CAD build for the part. Positions are in the model's coordinates, mm. Face numbers are marked on the shaded views. A direction names the side the tool comes from. Round coordinates to 2 decimals unless told otherwise and drop trailing zeros. Order: outer loops, then holes, each group sorted by start corner. A loop starts at its lowest first (then second) coordinate and runs counter-clockwise, first axis right, second up.
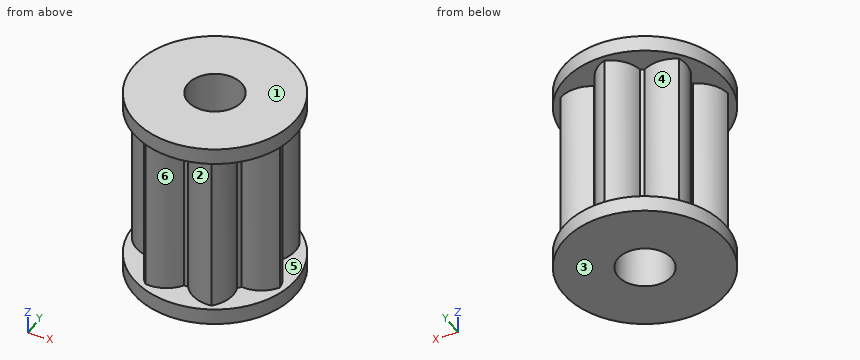
```python
from build123d import *

# Parameters (mm, degrees)
F0_R     = 2.5
F1_DEPTH = 15
F2_R     = 7.5
F2_R_2   = 2.5
F3_DEPTH = 1.5
F4_R     = 7.5
F4_R_2   = 2.5
F5_DEPTH = 1.5


with BuildPart() as f1:
    # F0 (on Top) → F1 (new body)
    with BuildSketch(Plane.XY):
        with BuildLine():
            ThreePointArc((0, 7), (-1.3412127701, 6.0735823287), (-2, 4.582575695))
            ThreePointArc((-2, 4.582575695), (-2.1694186956, 4.5048443395), (-2.3358223454, 4.420852177))
            ThreePointArc((-2.3358223454, 4.420852177), (-3.9122853917, 4.8354190111), (-5.4728203773, 4.364428613))
            ThreePointArc((-5.4728203773, 4.364428613), (-5.5847503602, 2.7382142744), (-4.8297815528, 1.2935262471))
            ThreePointArc((-4.8297815528, 1.2935262471), (-4.8746395609, 1.1126046698), (-4.9127228226, 0.9301368008))
            ThreePointArc((-4.9127228226, 0.9301368008), (-6.2197528574, -0.0439134465), (-6.8244953853, -1.5576465377))
            ThreePointArc((-6.8244953853, -1.5576465377), (-5.622857021, -2.659084978), (-4.0226390868, -2.9695748479))
            ThreePointArc((-4.0226390868, -2.9695748479), (-3.9091574123, -3.1174490093), (-3.7902428131, -3.2609905577))
            ThreePointArc((-3.7902428131, -3.2609905577), (-3.8436195617, -4.8901781832), (-3.0371861738, -6.3067820753))
            ThreePointArc((-3.0371861738, -6.3067820753), (-1.4268376596, -6.0540390065), (-0.1863673415, -4.9965255142))
            ThreePointArc((-0.1863673415, -4.9965255142), (0, -5), (0.1863673415, -4.9965255142))
            ThreePointArc((0.1863673415, -4.9965255142), (1.4268376596, -6.0540390065), (3.0371861738, -6.3067820753))
            ThreePointArc((3.0371861738, -6.3067820753), (3.8436195617, -4.8901781832), (3.7902428131, -3.2609905577))
            ThreePointArc((3.7902428131, -3.2609905577), (3.9091574123, -3.1174490093), (4.0226390868, -2.9695748479))
            ThreePointArc((4.0226390868, -2.9695748479), (5.622857021, -2.659084978), (6.8244953853, -1.5576465377))
            ThreePointArc((6.8244953853, -1.5576465377), (6.2197528574, -0.0439134465), (4.9127228226, 0.9301368008))
            ThreePointArc((4.9127228226, 0.9301368008), (4.8746395609, 1.1126046698), (4.8297815528, 1.2935262471))
            ThreePointArc((4.8297815528, 1.2935262471), (5.5847503602, 2.7382142744), (5.4728203773, 4.364428613))
            ThreePointArc((5.4728203773, 4.364428613), (3.9122853917, 4.8354190111), (2.3358223454, 4.420852177))
            ThreePointArc((2.3358223454, 4.420852177), (2.1694186956, 4.5048443395), (2, 4.582575695))
            ThreePointArc((2, 4.582575695), (1.3412127701, 6.0735823287), (0, 7))
        make_face()
        Circle(F0_R, mode=Mode.SUBTRACT)
    extrude(amount=F1_DEPTH)

    # F2 (on face) → F3 (join)
    with BuildSketch(Plane.XY.offset(15)):
        Circle(F2_R)
        with BuildLine():
            ThreePointArc((4.8297815528, 1.2935262471), (4.8746395609, 1.1126046698), (4.9127228226, 0.9301368008))
            ThreePointArc((4.9127228226, 0.9301368008), (6.2197528574, -0.0439134465), (6.8244953853, -1.5576465377))
            ThreePointArc((6.8244953853, -1.5576465377), (5.622857021, -2.659084978), (4.0226390868, -2.9695748479))
            ThreePointArc((4.0226390868, -2.9695748479), (3.9091574123, -3.1174490093), (3.7902428131, -3.2609905577))
            ThreePointArc((3.7902428131, -3.2609905577), (3.8436195617, -4.8901781832), (3.0371861738, -6.3067820753))
            ThreePointArc((3.0371861738, -6.3067820753), (1.4268376596, -6.0540390065), (0.1863673415, -4.9965255142))
            ThreePointArc((0.1863673415, -4.9965255142), (0, -5), (-0.1863673415, -4.9965255142))
            ThreePointArc((-0.1863673415, -4.9965255142), (-1.4268376596, -6.0540390065), (-3.0371861738, -6.3067820753))
            ThreePointArc((-3.0371861738, -6.3067820753), (-3.8436195617, -4.8901781832), (-3.7902428131, -3.2609905577))
            ThreePointArc((-3.7902428131, -3.2609905577), (-3.9091574123, -3.1174490093), (-4.0226390868, -2.9695748479))
            ThreePointArc((-4.0226390868, -2.9695748479), (-5.622857021, -2.659084978), (-6.8244953853, -1.5576465377))
            ThreePointArc((-6.8244953853, -1.5576465377), (-6.2197528574, -0.0439134465), (-4.9127228226, 0.9301368008))
            ThreePointArc((-4.9127228226, 0.9301368008), (-4.8746395609, 1.1126046698), (-4.8297815528, 1.2935262471))
            ThreePointArc((-4.8297815528, 1.2935262471), (-5.5847503602, 2.7382142744), (-5.4728203773, 4.364428613))
            ThreePointArc((-5.4728203773, 4.364428613), (-3.9122853917, 4.8354190111), (-2.3358223454, 4.420852177))
            ThreePointArc((-2.3358223454, 4.420852177), (-2.1694186956, 4.5048443395), (-2, 4.582575695))
            ThreePointArc((-2, 4.582575695), (-1.3412127701, 6.0735823287), (0, 7))
            ThreePointArc((0, 7), (1.3412127701, 6.0735823287), (2, 4.582575695))
            ThreePointArc((2, 4.582575695), (2.1694186956, 4.5048443395), (2.3358223454, 4.420852177))
            ThreePointArc((2.3358223454, 4.420852177), (3.9122853917, 4.8354190111), (5.4728203773, 4.364428613))
            ThreePointArc((5.4728203773, 4.364428613), (5.5847503602, 2.7382142744), (4.8297815528, 1.2935262471))
        make_face(mode=Mode.SUBTRACT)
        with BuildLine():
            ThreePointArc((6.8244953853, -1.5576465377), (6.2197528574, -0.0439134465), (4.9127228226, 0.9301368008))
            ThreePointArc((4.9127228226, 0.9301368008), (4.8746395609, 1.1126046698), (4.8297815528, 1.2935262471))
            ThreePointArc((4.8297815528, 1.2935262471), (5.5847503602, 2.7382142744), (5.4728203773, 4.364428613))
            ThreePointArc((5.4728203773, 4.364428613), (3.9122853917, 4.8354190111), (2.3358223454, 4.420852177))
            ThreePointArc((2.3358223454, 4.420852177), (2.1694186956, 4.5048443395), (2, 4.582575695))
            ThreePointArc((2, 4.582575695), (1.3412127701, 6.0735823287), (0, 7))
            ThreePointArc((0, 7), (-1.3412127701, 6.0735823287), (-2, 4.582575695))
            ThreePointArc((-2, 4.582575695), (-2.1694186956, 4.5048443395), (-2.3358223454, 4.420852177))
            ThreePointArc((-2.3358223454, 4.420852177), (-3.9122853917, 4.8354190111), (-5.4728203773, 4.364428613))
            ThreePointArc((-5.4728203773, 4.364428613), (-5.5847503602, 2.7382142744), (-4.8297815528, 1.2935262471))
            ThreePointArc((-4.8297815528, 1.2935262471), (-4.8746395609, 1.1126046698), (-4.9127228226, 0.9301368008))
            ThreePointArc((-4.9127228226, 0.9301368008), (-6.2197528574, -0.0439134465), (-6.8244953853, -1.5576465377))
            ThreePointArc((-6.8244953853, -1.5576465377), (-5.622857021, -2.659084978), (-4.0226390868, -2.9695748479))
            ThreePointArc((-4.0226390868, -2.9695748479), (-3.9091574123, -3.1174490093), (-3.7902428131, -3.2609905577))
            ThreePointArc((-3.7902428131, -3.2609905577), (-3.8436195617, -4.8901781832), (-3.0371861738, -6.3067820753))
            ThreePointArc((-3.0371861738, -6.3067820753), (-1.4268376596, -6.0540390065), (-0.1863673415, -4.9965255142))
            ThreePointArc((-0.1863673415, -4.9965255142), (0, -5), (0.1863673415, -4.9965255142))
            ThreePointArc((0.1863673415, -4.9965255142), (1.4268376596, -6.0540390065), (3.0371861738, -6.3067820753))
            ThreePointArc((3.0371861738, -6.3067820753), (3.8436195617, -4.8901781832), (3.7902428131, -3.2609905577))
            ThreePointArc((3.7902428131, -3.2609905577), (3.9091574123, -3.1174490093), (4.0226390868, -2.9695748479))
            ThreePointArc((4.0226390868, -2.9695748479), (5.622857021, -2.659084978), (6.8244953853, -1.5576465377))
        make_face()
        Circle(F2_R_2, mode=Mode.SUBTRACT)
    extrude(amount=F3_DEPTH)

    # F4 (on face) → F5 (join)
    with BuildSketch(Plane(origin=(0, 0, 0), x_dir=(1, 0, 0), z_dir=(0, 0, -1))):
        Circle(F4_R)
        with BuildLine():
            ThreePointArc((4.9127228226, -0.9301368008), (4.8746395609, -1.1126046698), (4.8297815528, -1.2935262471))
            ThreePointArc((4.8297815528, -1.2935262471), (5.5847503602, -2.7382142744), (5.4728203773, -4.364428613))
            ThreePointArc((5.4728203773, -4.364428613), (3.9122853917, -4.8354190111), (2.3358223454, -4.420852177))
            ThreePointArc((2.3358223454, -4.420852177), (2.1694186956, -4.5048443395), (2, -4.582575695))
            ThreePointArc((2, -4.582575695), (1.3412127701, -6.0735823287), (0, -7))
            ThreePointArc((0, -7), (-1.3412127701, -6.0735823287), (-2, -4.582575695))
            ThreePointArc((-2, -4.582575695), (-2.1694186956, -4.5048443395), (-2.3358223454, -4.420852177))
            ThreePointArc((-2.3358223454, -4.420852177), (-3.9122853917, -4.8354190111), (-5.4728203773, -4.364428613))
            ThreePointArc((-5.4728203773, -4.364428613), (-5.5847503602, -2.7382142744), (-4.8297815528, -1.2935262471))
            ThreePointArc((-4.8297815528, -1.2935262471), (-4.8746395609, -1.1126046698), (-4.9127228226, -0.9301368008))
            ThreePointArc((-4.9127228226, -0.9301368008), (-6.2197528574, 0.0439134465), (-6.8244953853, 1.5576465377))
            ThreePointArc((-6.8244953853, 1.5576465377), (-5.622857021, 2.659084978), (-4.0226390868, 2.9695748479))
            ThreePointArc((-4.0226390868, 2.9695748479), (-3.9091574123, 3.1174490093), (-3.7902428131, 3.2609905577))
            ThreePointArc((-3.7902428131, 3.2609905577), (-3.8436195617, 4.8901781832), (-3.0371861738, 6.3067820753))
            ThreePointArc((-3.0371861738, 6.3067820753), (-1.4268376596, 6.0540390065), (-0.1863673415, 4.9965255142))
            ThreePointArc((-0.1863673415, 4.9965255142), (0, 5), (0.1863673415, 4.9965255142))
            ThreePointArc((0.1863673415, 4.9965255142), (1.4268376596, 6.0540390065), (3.0371861738, 6.3067820753))
            ThreePointArc((3.0371861738, 6.3067820753), (3.8436195617, 4.8901781832), (3.7902428131, 3.2609905577))
            ThreePointArc((3.7902428131, 3.2609905577), (3.9091574123, 3.1174490093), (4.0226390868, 2.9695748479))
            ThreePointArc((4.0226390868, 2.9695748479), (5.622857021, 2.659084978), (6.8244953853, 1.5576465377))
            ThreePointArc((6.8244953853, 1.5576465377), (6.2197528574, 0.0439134465), (4.9127228226, -0.9301368008))
        make_face(mode=Mode.SUBTRACT)
        with BuildLine():
            ThreePointArc((5.4728203773, -4.364428613), (5.5847503602, -2.7382142744), (4.8297815528, -1.2935262471))
            ThreePointArc((4.8297815528, -1.2935262471), (4.8746395609, -1.1126046698), (4.9127228226, -0.9301368008))
            ThreePointArc((4.9127228226, -0.9301368008), (6.2197528574, 0.0439134465), (6.8244953853, 1.5576465377))
            ThreePointArc((6.8244953853, 1.5576465377), (5.622857021, 2.659084978), (4.0226390868, 2.9695748479))
            ThreePointArc((4.0226390868, 2.9695748479), (3.9091574123, 3.1174490093), (3.7902428131, 3.2609905577))
            ThreePointArc((3.7902428131, 3.2609905577), (3.8436195617, 4.8901781832), (3.0371861738, 6.3067820753))
            ThreePointArc((3.0371861738, 6.3067820753), (1.4268376596, 6.0540390065), (0.1863673415, 4.9965255142))
            ThreePointArc((0.1863673415, 4.9965255142), (0, 5), (-0.1863673415, 4.9965255142))
            ThreePointArc((-0.1863673415, 4.9965255142), (-1.4268376596, 6.0540390065), (-3.0371861738, 6.3067820753))
            ThreePointArc((-3.0371861738, 6.3067820753), (-3.8436195617, 4.8901781832), (-3.7902428131, 3.2609905577))
            ThreePointArc((-3.7902428131, 3.2609905577), (-3.9091574123, 3.1174490093), (-4.0226390868, 2.9695748479))
            ThreePointArc((-4.0226390868, 2.9695748479), (-5.622857021, 2.659084978), (-6.8244953853, 1.5576465377))
            ThreePointArc((-6.8244953853, 1.5576465377), (-6.2197528574, 0.0439134465), (-4.9127228226, -0.9301368008))
            ThreePointArc((-4.9127228226, -0.9301368008), (-4.8746395609, -1.1126046698), (-4.8297815528, -1.2935262471))
            ThreePointArc((-4.8297815528, -1.2935262471), (-5.5847503602, -2.7382142744), (-5.4728203773, -4.364428613))
            ThreePointArc((-5.4728203773, -4.364428613), (-3.9122853917, -4.8354190111), (-2.3358223454, -4.420852177))
            ThreePointArc((-2.3358223454, -4.420852177), (-2.1694186956, -4.5048443395), (-2, -4.582575695))
            ThreePointArc((-2, -4.582575695), (-1.3412127701, -6.0735823287), (0, -7))
            ThreePointArc((0, -7), (1.3412127701, -6.0735823287), (2, -4.582575695))
            ThreePointArc((2, -4.582575695), (2.1694186956, -4.5048443395), (2.3358223454, -4.420852177))
            ThreePointArc((2.3358223454, -4.420852177), (3.9122853917, -4.8354190111), (5.4728203773, -4.364428613))
        make_face()
        Circle(F4_R_2, mode=Mode.SUBTRACT)
    extrude(amount=F5_DEPTH)


solid = f1.part
```
1. Tool access for the marked faces 4, 5 and 6: list every direction of +Z, -Z, +X, -X, +Y, -Y with a clear straight run to the whole face (end or side of a thin tool).
2. Drill centre lines: line 1 (Z direction, x = -4.5, y = -4.25); line 2 (Y direction, x = 0, z = 12.5); line 3 (Y direction, x = 0, z = 15.5). Where is each one in solid material? Low to high.
3. Pin check, flat tips, straight feed: P1, Ø5, axis at y = 2.5, z = 13, coming from the +X side; P2, Ø3, axis at x = -3, z = 7, coming from the -Y side; P3, Ø1.5, axis at y = 2.5, z = 3.5, coming from the -X side. Stop position of each tip, or through.
4. Cut at A-A, the plane z = 3.5. Write the cut outline in (x, y), and give its area (3 significant figures).
5. Mould opens along Z. For the marked faces 1, 2 and 3 say: released by +Z, released by -Z, zero draft, split by the parting line, or undercut.
6. Cut at D-D, the plane x = -2.75. Write the cut outline in (y, z).
7. Cut at B-B, the plane x = 1.5. Write the cut outline in (y, z).
8. Cut at C-C, the plane y = 0. Write the cut outline in (x, z).
Outcome:
1. face 4: +Y
1. face 5: none
1. face 6: -Y
2. line 1: z = -1.5 to 0, 15 to 16.5
2. line 2: y = -5 to -2.5, 2.5 to 7
2. line 3: y = -7.5 to -2.5, 2.5 to 7.5
3. P1: stops at x = 7.43
3. P2: stops at y = -6.33
3. P3: stops at x = -5.65
4. outline: (-6.82, -1.56) arc R3 ccw to (-4.02, -2.97) arc R5 ccw to (-3.79, -3.26) arc R3 ccw to (-3.04, -6.31) arc R3 ccw to (-0.19, -5) arc R5 ccw to (0.19, -5) arc R3 ccw to (3.04, -6.31) arc R3 ccw to (3.79, -3.26) arc R5 ccw to (4.02, -2.97) arc R3 ccw to (6.82, -1.56) arc R3 ccw to (4.91, 0.93) arc R5 ccw to (4.83, 1.29) arc R3 ccw to (5.47, 4.36) arc R3 ccw to (2.34, 4.42) arc R5 ccw to (2, 4.58) arc R3 ccw to (0, 7) arc R3 ccw to (-2, 4.58) arc R5 ccw to (-2.34, 4.42) arc R3 ccw to (-5.47, 4.36) arc R3 ccw to (-4.83, 1.29) arc R5 ccw to (-4.91, 0.93) arc R3 ccw to start; hole circle Ø5 at (0, 0)
4. area: 98.1 mm2
5. face 1: released by +Z
5. face 2: undercut
5. face 3: released by -Z
6. outline: (-6.98, -1.5) - (6.98, -1.5) - (6.98, 0) - (4.62, 0) - (4.62, 15) - (6.98, 15) - (6.98, 16.5) - (-6.98, 16.5) - (-6.98, 15) - (-6.33, 15) - (-6.33, 0) - (-6.98, 0) - close
7. outline: (-7.35, -1.5) - (-2, -1.5) - (-2, 16.5) - (-7.35, 16.5) - (-7.35, 15) - (-6.09, 15) - (-6.09, 0) - (-7.35, 0) - close; (2, -1.5) - (7.35, -1.5) - (7.35, 0) - (5.86, 0) - (5.86, 15) - (7.35, 15) - (7.35, 16.5) - (2, 16.5) - close
8. outline: (-7.5, -1.5) - (-2.5, -1.5) - (-2.5, 16.5) - (-7.5, 16.5) - (-7.5, 15) - (-6.19, 15) - (-6.19, 0) - (-7.5, 0) - close; (2.5, -1.5) - (7.5, -1.5) - (7.5, 0) - (6.19, 0) - (6.19, 15) - (7.5, 15) - (7.5, 16.5) - (2.5, 16.5) - close
